Job drawing, mm, ordinate dimensions from the low corner. One solid piece. A direction names the side the tool comes from. Give positions to 0.01 mm unless a question says otherwise; leave off trailing zeros. Order: outer loops, then holes, each group sorted by start corner. A loop starts at its lowest first (then second) coordinate and runs counter-clockwise, first axis right, second up.
1. Which spindle directions (+Z, -Z, +X, -X, +Y, -Y) get a long thin tool onto all of the face, cutting with end or side? Do the marked faces 1, 2, 3 and 4. Say none if no direction does.
2. Slice it at A-A on z = 19.05. Give the number of separate pieces and of enclosed holes in the cut face, and give its area (3 significant figures).
3. Drop flat-ended pins along their axis: pin 1 Ø1 at (x, z) = (5, 26) entering from +Y; pin 2 Ø3 at (x, y) = (3, 46) entering from -Z; pin 3 Ø1.9 at (x, z) = (2, 7) entering from -Y; pin 4 Ø3 at (y, z) = (3.175, 19.05) entering from -X. Give the stop position or say it passes through.
4. Slice it at B-B on y = 28. List the corners of the cut face in (x, z).
5. Mould opens along Z. For the marked faces 5, 6, 7 and 8 say: +Z half, -Z half, draft (parallel to the pull), parting line (faces both ways), or undercut.
6. Slice it at D-D on z = 26. List the corners of the cut face in (x, y).
7. Probe line 1 (Y direction, x = 2, z = 19.05) (1 decimal); line 2 (Y direction, x = 4.75, z = 10.5); line 3 (Z direction, x = 1.75, y = 28) (1 decimal). List the from-to ranges inside material, lowest first.
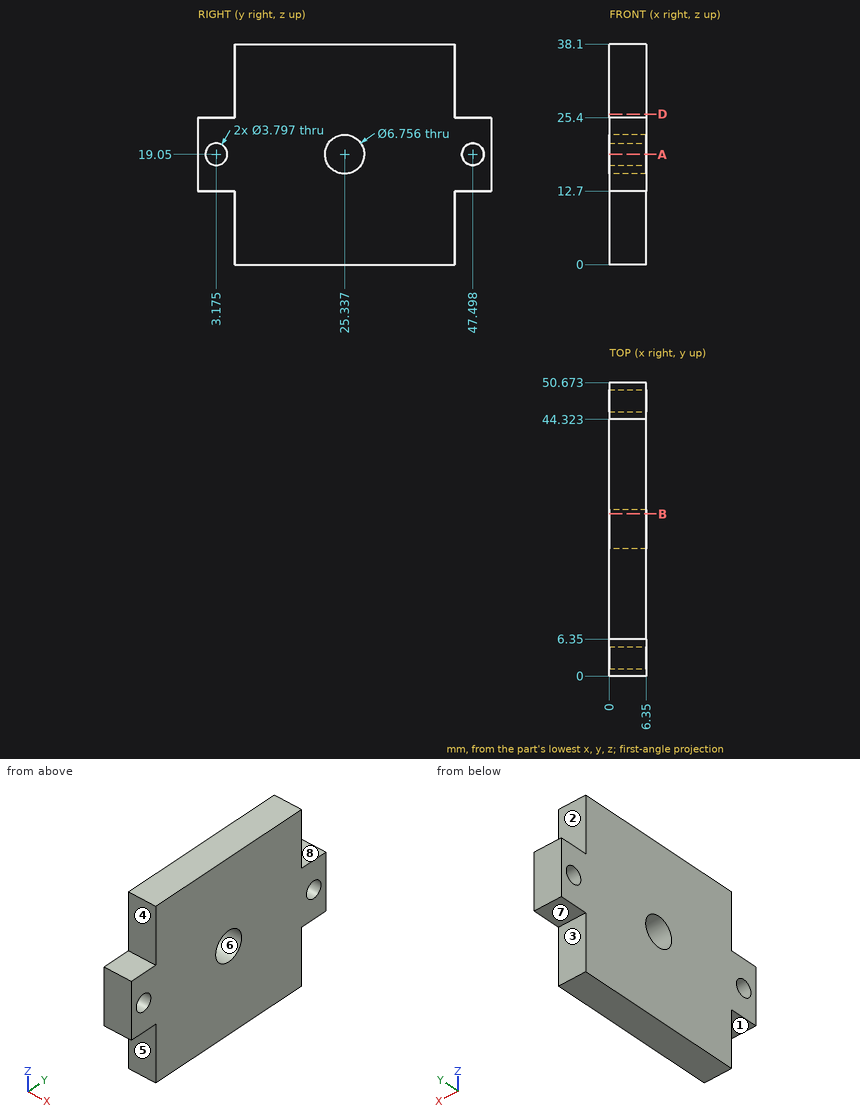
Data:
1. face 1: -Z, +X, -X, -Y
1. face 2: +Z, +X, -X, +Y
1. face 3: -Z, +X, -X, +Y
1. face 4: +Z, +X, -X, -Y
2. separate pieces: 4
2. enclosed holes: 0
2. area: 231 mm2
3. pin 1: stops at y = 44.32
3. pin 2: stops at z = 12.7
3. pin 3: stops at y = 6.35
3. pin 4: passes through
4. outline: (0, 0) - (6.35, 0) - (6.35, 16.97) - (0, 16.97) - close; (0, 21.13) - (6.35, 21.13) - (6.35, 38.1) - (0, 38.1) - close
5. face 5: draft
5. face 6: undercut
5. face 7: -Z half
5. face 8: +Z half
6. outline: (0, 6.35) - (6.35, 6.35) - (6.35, 44.32) - (0, 44.32) - close
7. line 1: y = 0 to 1.3, 5.1 to 22, 28.7 to 45.6, 49.4 to 50.7
7. line 2: y = 6.35 to 44.32
7. line 3: z = 0 to 17, 21.1 to 38.1
